Here's the drawing with two shaded views (mm, measured from the low corner). I have some questions. Coordinates: 2 decimals unless noted, no trailing zeros. Loops run counter-clockwise (first coordinate to the right, second up) from the corner with the lowest first, then second, coordinate; pieces in that order, holes last.
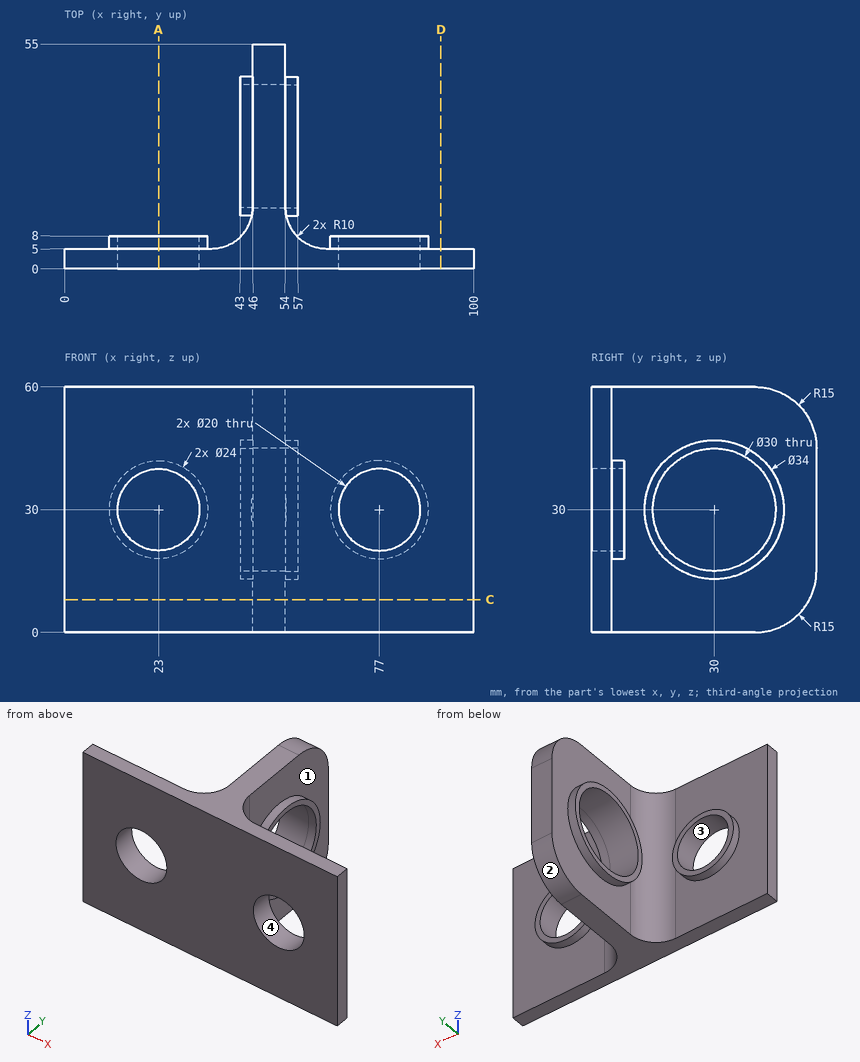
Q1. Suppose I cut it at A-A on x = 23. Write out the boundary of the cut face in (y, z).
Q2. Suppose I cut it at D-D on x = 92. Write out the boundary of the cut face in (y, z).
Q3. Will these pins go through, and if not, where does the flat tip stop? P1, Ø4, axis at x = 42.5, y = 28.5, coming from the -Z side; P2, Ø11, axis at x = 14.5, z = 37.5, coming from the +Y side; P3, Ø3, axis at y = 22.5, z = 7.5, coming from the +X side.
Q4. We'd pull the mould along X, two halves only. Please class the marked faces 1, 2, 3 and 4: pulls with the +X half, pulls with the -X half, needs draft (parallel to the pull), parting line crosses it, or undercut.
Q5. Please list where these lines run through material, in increasing order: probe 1 along X at (y, z) = (4, 30); probe 2 along Z at (x, y) = (77, 2.5); probe 3 along Y at (x, z) = (46.5, 39).
Q6. Suppose I cut it at C-C on z = 8. Write out the boundary of the cut face in (x, y), and give its area (3 significant figures).
Check values:
1. outline: (0, 0) - (5, 0) - (5, 18) - (8, 18) - (8, 20) - (0, 20) - close; (0, 40) - (8, 40) - (8, 42) - (5, 42) - (5, 60) - (0, 60) - close
2. outline: (0, 0) - (5, 0) - (5, 60) - (0, 60) - close
3. P1: stops at z = 13
3. P2: stops at y = 8
3. P3: stops at x = 54
4. face 1: pulls with the +X half
4. face 2: needs draft
4. face 3: undercut
4. face 4: undercut
5. probe 1: x = 0 to 13, 33 to 67, 87 to 100
5. probe 2: z = 0 to 20, 40 to 60
5. probe 3: y = 0 to 18, 42 to 55
6. outline: (0, 0) - (100, 0) - (100, 5) - (64, 5) arc R10 cw to (54, 15) - (54, 53.27) - (46, 53.27) - (46, 15) arc R10 cw to (36, 5) - (0, 5) - close
6. area: 929 mm2
